For this review, take the finished solid that the model builds, in its own axes (mm). Face numbers are marked on the shaded views. A direction names the side the tool comes from. Coordinates: 2 decimals unless noted, no trailing zeros. Loops run counter-clockwise (first coordinate to the right, second up) from the corner with the lowest first, then second, coordinate; pieces in that order, holes last.
1. Clearance check with flat-ended pins moving along their axes: P1, Ø5, axis at x = -2, y = 12.5, coming from the +Z side; P2, Ø4, axis at x = 31.18, z = 18, coming from the +Y side; P3, Ø2.5, axis at x = 0, z = -36, coming from the +Y side; P4, Ø3, axis at y = 36, z = -49, coming from the +X side. State where each tip first meets the part, or that it passes through.
2. To check wall thickness, follow probe 1 along Z at (x, y) = (0, 3); probe 2 along Y at (x, z) = (-28.5, 19); probe 3 along Y at (x, z) = (-5, 0.5). State the ranges of each line that lie inside material, in increasing order.
3. Take a section at C-C, the plane z = -36. State the section outline as (x, y) points.
4. Machinability: for the marked faces 1, 2 and 3, which of the approach directions +Z, -Z, +X, -X, +Y, -Y give a long, thin tool a straight path to every point of the face, cutting with its end or side? Answer none if there is none.
5. Take a section at A-A, the plane x = 0. State the section outline as (y, z) points.
6. Take a section at D-D, the plane x = 24. State the section outline as (y, z) points.
7. Take a section at B-B, the plane z = 18. State the section outline as (x, y) points, then the cut area to 3 significant figures.
```python
from build123d import *

# Parameters (mm, degrees)
SKETCH1_R           = 40
BOSS_EXTRUDE1_DEPTH = 6
SKETCH2_R           = 1.5
BOSS_EXTRUDE2_DEPTH = 2
SKETCH16_R          = 1.5
CUT_EXTRUDE9_DEPTH  = 9
CIRPATTERN1_COUNT   = 3
SKETCH5_R           = 30.471270003
CUT_EXTRUDE3_DEPTH  = 7
CIRPATTERN2_COUNT   = 3
BOSS_EXTRUDE3_DEPTH = 6
SKETCH18_W          = 33.849231786
SKETCH18_H          = 60
BOSS_EXTRUDE4_DEPTH = 4
CHAMFER1_SIZE       = 2
SKETCH19_W          = 22
SKETCH19_H          = 10
CUT_EXTRUDE10_DEPTH = 25
FILLET1_R           = 4
FILLET2_R           = 10


with BuildPart() as part:
    # Sketch1 → Boss-Extrude1 (new body)
    with BuildSketch(Plane(origin=(0, 0, 0), x_dir=(1, 0, 0), z_dir=(0, 1, 0))):
        Circle(SKETCH1_R)
    extrude(amount=BOSS_EXTRUDE1_DEPTH)

    # Sketch2 → Boss-Extrude2 (add)
    with BuildSketch(Plane(origin=(0, 6, 0), x_dir=(1, 0, 0), z_dir=(0, 1, 0))):
        with BuildLine():
            Line((-13.680805733, 37.587704831), (-10.944644586, 30.070163865))
            ThreePointArc((-10.944644586, 30.070163865), (0, 32), (10.944644586, 30.070163865))
            Line((10.944644586, 30.070163865), (13.680805733, 37.587704831))
            ThreePointArc((13.680805733, 37.587704831), (0, 40), (-13.680805733, 37.587704831))
        make_face()
        with Locations((0, 36)):
            Circle(SKETCH2_R, mode=Mode.SUBTRACT)
    boss_extrude2 = extrude(amount=BOSS_EXTRUDE2_DEPTH)

    # Sketch16 → Cut-Extrude9 (cut, through all)
    with BuildSketch(Plane(origin=(0, 8, 0), x_dir=(1, 0, 0), z_dir=(0, 1, 0))):
        with Locations((0, 36)):
            Circle(SKETCH16_R)
    cut_extrude9 = extrude(amount=-CUT_EXTRUDE9_DEPTH, mode=Mode.SUBTRACT)

    # CirPattern1: Boss-Extrude2, Cut-Extrude9 ×3 about axis
    cirpattern1_axis = Axis((0, 0, 0), (0, 1, 0))
    for i in range(1, CIRPATTERN1_COUNT):
        add(boss_extrude2.rotate(cirpattern1_axis, i * 360 / CIRPATTERN1_COUNT))
        add(cut_extrude9.rotate(cirpattern1_axis, i * 360 / CIRPATTERN1_COUNT), mode=Mode.SUBTRACT)

    # Sketch5 → Cut-Extrude3 (cut, through all)
    with BuildSketch(Plane(origin=(0, 6, 0), x_dir=(1, 0, 0), z_dir=(0, 1, 0))):
        with Locations((40.698571494, 23.497331208)):
            Circle(SKETCH5_R)
    cut_extrude3 = extrude(amount=-CUT_EXTRUDE3_DEPTH, mode=Mode.SUBTRACT)

    # CirPattern2: Cut-Extrude3 ×3 about axis
    cirpattern2_axis = Axis((0, 0, 0), (0, 1, 0))
    for i in range(1, CIRPATTERN2_COUNT):
        add(cut_extrude3.rotate(cirpattern2_axis, i * 360 / CIRPATTERN2_COUNT), mode=Mode.SUBTRACT)

    # Sketch17 → Boss-Extrude3 (add)
    with BuildSketch(Plane(origin=(0, 0, 0), x_dir=(1, 0, 0), z_dir=(0, 1, 0))):
        with BuildLine():
            Line((-13.680805733, 37.587704831), (-16.924615893, 46.5))
            Line((-16.924615893, 46.5), (16.924615893, 46.5))
            Line((16.924615893, 46.5), (13.680805733, 37.587704831))
            ThreePointArc((13.680805733, 37.587704831), (0, 40), (-13.680805733, 37.587704831))
        make_face()
    extrude(amount=BOSS_EXTRUDE3_DEPTH)

    # Sketch18 → Boss-Extrude4 (add)
    with BuildSketch(Plane(origin=(0, 0, -46.5), x_dir=(-1, 0, 0), z_dir=(0, 0, -1))):
        with Locations((0, 30)):
            Rectangle(SKETCH18_W, SKETCH18_H)
    extrude(amount=BOSS_EXTRUDE4_DEPTH)

    # Chamfer1
    chamfer1_edges = [part.edges().sort_by_distance(p)[0] for p in [
        (0, 6, -46.5),
    ]]
    chamfer(chamfer1_edges, length=CHAMFER1_SIZE)

    # Sketch19 → Cut-Extrude10 (cut)
    with BuildSketch(Plane(origin=(0, 6, 0), x_dir=(1, 0, 0), z_dir=(0, 1, 0))):
        with Locations((0, -15.5)):
            Rectangle(SKETCH19_W, SKETCH19_H)
    extrude(amount=-CUT_EXTRUDE10_DEPTH, mode=Mode.SUBTRACT)

    # Fillet1
    fillet1_edges = [part.edges().sort_by_distance(p)[0] for p in [
        (-11, 3, 18.578147929),
        (11, 3, 18.578147929),
        (-11, 3, 10.5),
        (11, 3, 10.5),
    ]]
    fillet(fillet1_edges, radius=FILLET1_R)

    # Fillet2
    fillet2_edges = [part.edges().sort_by_distance(p)[0] for p in [
        (16.924615893, 60, -48.5),
        (-16.924615893, 60, -48.5),
    ]]
    fillet(fillet2_edges, radius=FILLET2_R)


solid = part.part
```
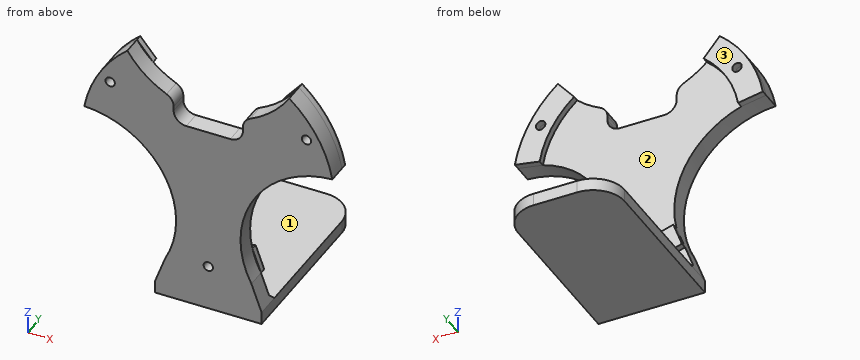
Results list:
1. P1: stops at z = -46.5
1. P2: stops at y = 8
1. P3: passes through
1. P4: stops at x = 16.92
2. probe 1: z = -50.5 to -37.5, -34.5 to 10.5
2. probe 2: y = 0 to 8
2. probe 3: y = 0 to 6
3. outline: (-13.1, 6) - (-12.91, 6) - (-12.91, 0) - (-1.5, 0) - (-1.5, 8) - (-13.1, 8) - close; (1.5, 0) - (12.91, 0) - (12.91, 6) - (13.1, 6) - (13.1, 8) - (1.5, 8) - close
4. face 1: +Z, +X, -X, +Y
4. face 2: +Y
4. face 3: +Z, -Z, +X, -X, +Y
5. outline: (0, -50.5) - (60, -50.5) - (60, -46.5) - (8, -46.5) - (6, -44.5) - (6, -40) - (8, -40) - (8, -37.5) - (0, -37.5) - close; (0, -34.5) - (8, -34.5) - (8, -32) - (6, -32) - (6, 10.5) - (0, 10.5) - close
6. outline: (0, 1.99) - (6, 1.99) - (6, 21.17) - (8, 21.17) - (8, 28.6) - (6, 28.6) - (6, 28.22) - (0, 28.22) - close
7. outline: (-35.72, 0) - (-32.68, 0) - (-32.68, 8) - (-35.72, 8) - close; (-29.68, 0) - (-11.56, 0) - (-11.56, 6) - (-26.46, 6) - (-26.46, 8) - (-29.68, 8) - close; (11.56, 0) - (29.68, 0) - (29.68, 8) - (26.46, 8) - (26.46, 6) - (11.56, 6) - close; (32.68, 0) - (35.72, 0) - (35.72, 8) - (32.68, 8) - close
7. area: 279 mm2
